Design review of the part built by this model. Coordinates are the model's own, in mm. Face numbers are marked on the shaded views. A direction names the side the tool comes from. Coordinates: 2 decimals unless noted, no trailing zeros. Write each loop counter-clockwise with the first axis right and the second up, starting at its lowest first coordinate (ties: lowest second). Pieces come first, ordered by that corner, then holes.
Q1. The part is to be moulded in two halves that separate along Y. For the marked faces 3, 4 and 5, say which applies: +Y half, -Y half, draft (parallel to the pull), parting line (faces both ways), or undercut.
Q2. Add section A-A, the plane y = 22. Give the boundary of the cut face in (x, z), plus the area to 3 significant figures.
Q3. Add section D-D, the plane y = 42. Give the boundary of the cut face in (x, z), plus the area to 3 significant figures.
Q4. Machinability: for the marked faces 1 and 2, which of the approach directions +Z, -Z, +X, -X, +Y, -Y give a long, thin tool a straight path to every point of the face, cutting with its end or side? Answer none if there is none.
Q5. Add section B-B, the plane x = 53. Give the boundary of the cut face in (y, z), plus the area to 3 significant figures.
Q6. Add section C-C, the plane z = 1.25. Give the boundary of the cut face in (x, y), plus the area to 3 significant figures.
Q7. To check wall thickness, follow probe 1 along Y at (x, z) = (-10.5, -4); probe 2 along X at (y, z) = (48, -5.25); probe 3 along Y at (x, z) = (5.5, 0.25). State the ranges of each line that lie inside material, in increasing order.
Q8. Clearance check with flat-ended pins moving along their axes: pin 1 Ø2 at (x, y) = (31.5, 47) entering from -Z; pin 2 Ø10 at (x, y) = (54, 12.5) entering from +Z. State where each tip first meets the part, or that it passes through.
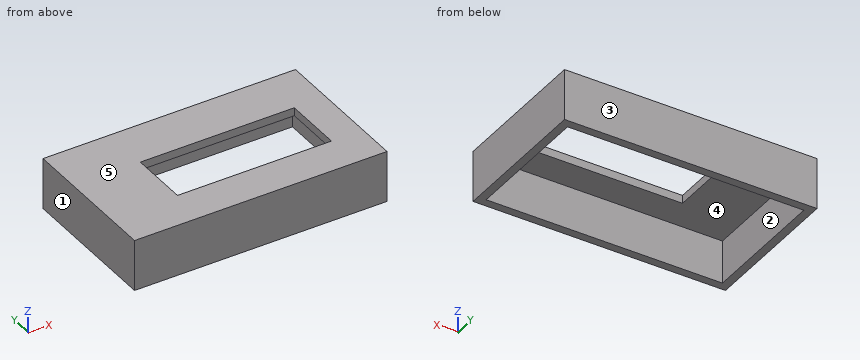
from build123d import *

# Parameters (mm, degrees)
SKETCH1_W           = 119.105009205
SKETCH1_H           = 68.796475466
SKETCH1_W_2         = 72.644
SKETCH1_H_2         = 27.94
BOSS_EXTRUDE2_DEPTH = 3.81
SKETCH2_W           = 119.105009205
SKETCH2_H           = 68.796475466
SKETCH2_W_2         = 111.485009205
SKETCH2_H_2         = 61.176475466
BOSS_EXTRUDE3_DEPTH = 20.32


with BuildPart() as part:
    # Sketch1 → Boss-Extrude2 (new body)
    with BuildSketch(Plane.XY):
        with Locations((32.019529699, 19.90260555)):
            Rectangle(SKETCH1_W, SKETCH1_H)
        with Locations((40.386, 17.526)):
            Rectangle(SKETCH1_W_2, SKETCH1_H_2, mode=Mode.SUBTRACT)
    extrude(amount=BOSS_EXTRUDE2_DEPTH)

    # Sketch2 → Boss-Extrude3 (add)
    with BuildSketch(Plane.XY):
        with Locations((32.019529699, 19.90260555)):
            Rectangle(SKETCH2_W, SKETCH2_H)
        with Locations((32.019529699, 19.90260555)):
            Rectangle(SKETCH2_W_2, SKETCH2_H_2, mode=Mode.SUBTRACT)
    extrude(amount=-BOSS_EXTRUDE3_DEPTH)


solid = part.part
Here are the results:
1. face 3: +Y half
1. face 4: undercut
1. face 5: draft
2. outline: (-27.53, -20.32) - (-23.72, -20.32) - (-23.72, 0) - (4.06, 0) - (4.06, 3.81) - (-27.53, 3.81) - close; (76.71, 0) - (87.76, 0) - (87.76, -20.32) - (91.57, -20.32) - (91.57, 3.81) - (76.71, 3.81) - close
2. area: 332 mm2
3. outline: (-27.53, -20.32) - (-23.72, -20.32) - (-23.72, 0) - (87.76, 0) - (87.76, -20.32) - (91.57, -20.32) - (91.57, 3.81) - (-27.53, 3.81) - close
3. area: 609 mm2
4. face 1: +Z, -Z, -X, +Y, -Y
4. face 2: -Z
5. outline: (-14.5, -20.32) - (-10.69, -20.32) - (-10.69, 0) - (3.56, 0) - (3.56, 3.81) - (-14.5, 3.81) - close; (31.5, 0) - (50.49, 0) - (50.49, -20.32) - (54.3, -20.32) - (54.3, 3.81) - (31.5, 3.81) - close
5. area: 311 mm2
6. outline: (-27.53, -14.5) - (91.57, -14.5) - (91.57, 54.3) - (-27.53, 54.3) - close; hole (4.06, 3.56) - (76.71, 3.56) - (76.71, 31.5) - (4.06, 31.5) - close
6. area: 6,160 mm2
7. probe 1: y = -14.5 to -10.69, 50.49 to 54.3
7. probe 2: x = -27.53 to -23.72, 87.76 to 91.57
7. probe 3: y = -14.5 to 3.56, 31.5 to 54.3
8. pin 1: stops at z = 0
8. pin 2: passes through
